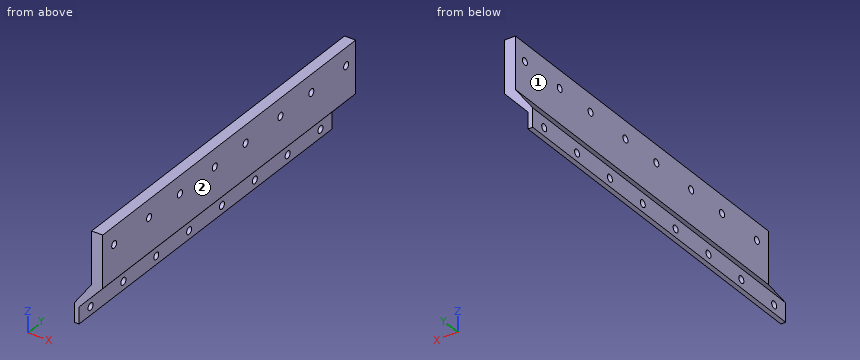
Autodesk Inventor part; units mm, degrees
ref_plane "YZ Plane" through (0, 0, 0) normal (1, 0, 0) x (0, 1, 0)
ref_plane "XZ Plane" through (0, 0, 0) normal (0, 1, 0) x (-1, 0, 0)
ref_plane "XY Plane" through (0, 0, 0) normal (0, 0, 1) x (1, 0, 0)
sketch "Sketch1" plane through (0, 0, 0) normal (0, 1, 0) x (-1, 0, 0)
  line L0 (0, 0) -> (-19.05, 0) construction
  line L1 (-19.05, 0) -> (-19.05, -19.05) construction
  line L2 (-19.05, -19.05) -> (0, -19.05) construction
  line L3 (0, -19.05) -> (0, 0) construction
  line L4 (0, 0) -> (279.4, 0) construction
  line L5 (279.4, 0) -> (279.4, -35.5) construction
  line L6 (279.4, -35.5) -> (0, -35.5) construction
  line L7 (0, -35.5) -> (0, 0) construction
  line L8 (-47.8536, 0) -> (-47.8536, -76.2) construction
  line L9 (-19.05, 0) -> (-24.9936, 0)
  line L10 (-24.9936, 0) -> (-24.9936, -27.94)
  line L11 (-24.9936, -27.94) -> (-19.05, -27.94)
  line L12 (-19.05, -27.94) -> (-19.05, 0)
  line L13 (-9.7536, -51) -> (-12.2936, -51)
  line L14 (-12.2936, -51) -> (-12.2936, -42.11)
  line L15 (-9.7536, -40.84) -> (-9.7536, -51)
  line L16 (-9.7536, -40.84) -> (-19.05, -27.94)
  line L17 (-9.7536, -42.11) -> (-12.2936, -42.11) construction
  line L18 (-12.2936, -42.11) -> (-24.9936, -27.94)
  dimension "d0" = 19.05
  dimension "d1" = 19.05
  dimension "d2" = 279.4
  dimension "d3" = 35.5
  dimension "d4" = 76.2
  dimension "d5" = 28.8036
  dimension "d6" = 38.1
  dimension "d7" = 51
  dimension "d8" = 5.9436
  dimension "d9" = 27.94
  dimension "d12" = 8.89
extrude "Extrusion1" add sketch "Sketch1" along normal blind 195.58
sketch "Sketch2" plane through (24.9936, 0, 0) normal (1, 0, 0) x (0, 0, -1)
  circle A0 centre (9.525, 8.89) radius 1.9304
  circle A1 centre (9.525, 35.8394) radius 1.9304
  line L0 (0, 0) -> (27.94, 0)
  line L1 (0, 0) -> (0, 195.58)
  circle A2 centre (9.525, 86.6394) radius 1.9304
  circle A3 centre (9.525, 59.69) radius 1.9304
  circle A4 centre (9.525, 137.4394) radius 1.9304
  circle A5 centre (9.525, 110.49) radius 1.9304
  circle A6 centre (9.525, 188.2394) radius 1.9304
  circle A7 centre (9.525, 161.29) radius 1.9304
  dimension "d16" = 3.8608
  dimension "d17" = 3.8608
  dimension "d18" = 26.9494
  dimension "d19" = 8.89
  dimension "d20" = 9.525
  dimension "d21" = 9.525
  dimension "d24" = 50.8
extrude "Extrusion2" cut sketch "Sketch2" against normal blind 195.58
sketch "Sketch3" plane through (9.7536, 0, -51) normal (-1, 0, 0) x (0, 0, 1)
  circle A0 centre (4.445, 8.89) radius 1.9304
  line L0 (0, 0) -> (0, 195.58)
  line L1 (0, 0) -> (10.16, 0)
  circle A1 centre (4.445, 34.29) radius 1.9304
  circle A2 centre (4.445, 59.69) radius 1.9304
  circle A3 centre (4.445, 85.09) radius 1.9304
  circle A4 centre (4.445, 110.49) radius 1.9304
  circle A5 centre (4.445, 135.89) radius 1.9304
  circle A6 centre (4.445, 161.29) radius 1.9304
  circle A7 centre (4.445, 186.69) radius 1.9304
  point P0 (51, 0)
  dimension "d31" = 3.8608
  dimension "d32" = 4.445
  dimension "d33" = 8.89
  dimension "d36" = 25.4
extrude "Extrusion3" cut sketch "Sketch3" against normal through all
equation "\"d21\" = d20"
properties part number "intake guide mount"
Source: CAD feature listing. Evaluate the final solid. Frame: model axes, mm. Face numbers are marked on the shaded views. A direction names the side the tool comes from. Round coordinates to 2 decimals unless told otherwise and drop trailing zeros. Write each loop counter-clockwise with the first axis right and the second up, starting at its lowest first coordinate (ties: lowest second). Pieces come first, ordered by that corner, then holes. Notation, with made-up numbers: M 76,18 L 116,18 A14 cw 116,26 Z; hole C 30.5,83.5 d1. An arc over 180 degrees is marked long. Use CSV: the item, a comma, the result in double quotes. Start each with the question number.
Q1. Access query for the marked faces 1 and 2. Directions: +Z, -Z, +X, -X, +Y, -Y. A direction counts if a zero-diameter tool reaches every point of the face in a straight line with its end or side. Return the directions, or none.
Q2. Line query: line 1 (X direction, y = 52, z = -46.5); line 2 (Z direction, x = 21.5, y = 110.5); line 3 (X direction, y = 101.5, z = -6). Output: solid intervals per line, ascending. Write a range as from..to.
Q3. Cut plane A-A on y = 59.69. Output: boundary loops of the cut face in (x, z), plus the area to 3 significant figures.
Q4. Cut plane C-C on x = 14.25. Output: boundary loops of the cut face in (y, z).
Q5. First-contact query: P1, Ø8, axis at y = 82.5, z = -16.5, coming from the -X side; P2, Ø5, axis at y = 34.29, z = -46.555, coming from the +X side; P3, Ø4, axis at y = 65.5, z = -35.5, coming from the +X side. Flat tips, straight axial feed; report the tip coordinate or a pass-through.
Q6. Cut plane B-B on y = 142. Output: boundary loops of the cut face in (x, z), plus the area to 3 significant figures.
Results found:
1,face 1,"+Z, -X, +Y, -Y"
1,face 2,"+Z, -Z, +X, +Y, -Y"
2,line 1,"9.75..12.29"
2,line 2,"-31.84..-11.46, -7.59..0"
2,line 3,"19.05..24.99"
3,outline,"M 9.75,-51 L 12.29,-51 L 12.29,-48.49 L 9.75,-48.49 Z; M 9.75,-44.62 L 12.29,-44.62 L 12.29,-42.11 L 24.99,-27.94 L 24.99,-11.46 L 19.05,-11.46 L 19.05,-27.94 L 9.75,-40.84 Z; M 19.05,-7.59 L 24.99,-7.59 L 24.99,0 L 19.05,0 Z"
3,area,"222 mm^2"
4,outline,"M 0,-39.93 L 195.58,-39.93 L 195.58,-34.6 L 0,-34.6 Z"
5,P1,"x = 19.05"
5,P2,"x = 12.29"
5,P3,"x = 20.01"
6,outline,"M 9.75,-51 L 12.29,-51 L 12.29,-42.11 L 24.99,-27.94 L 24.99,0 L 19.05,0 L 19.05,-27.94 L 9.75,-40.84 Z"
6,area,"255 mm^2"
